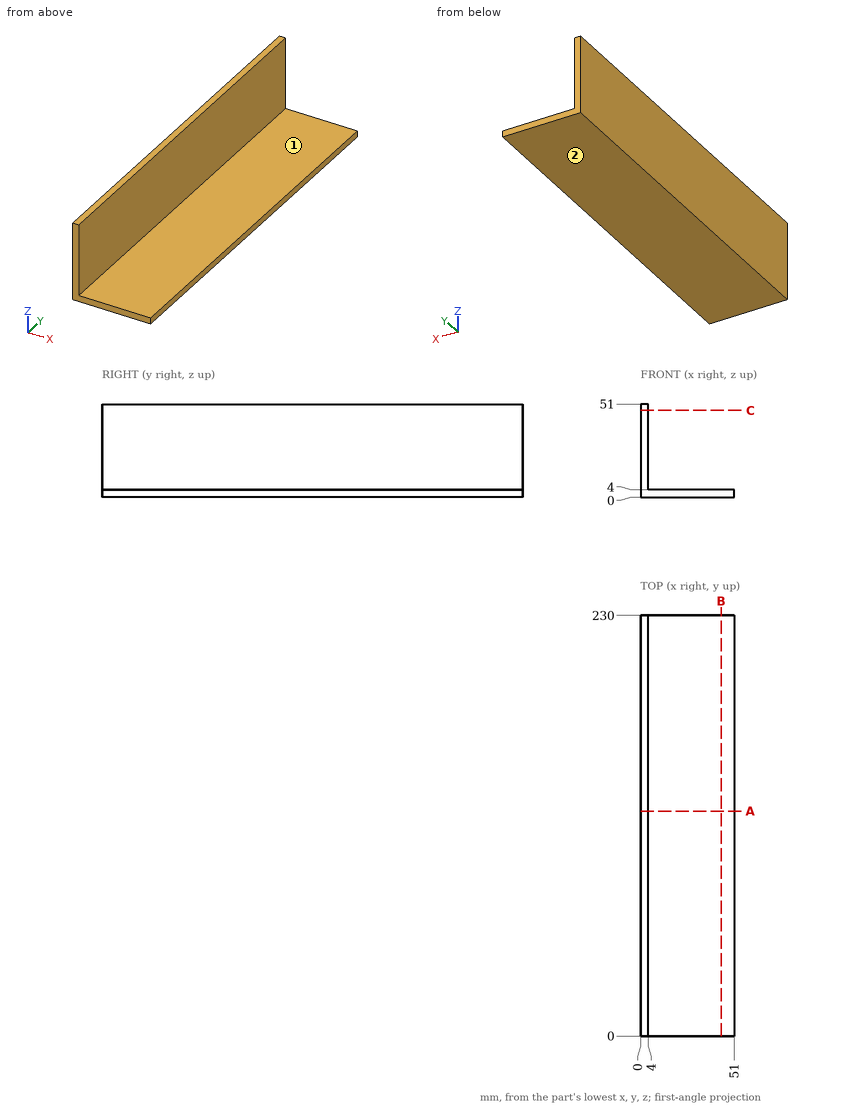
Study the drawing (mm; zero at the part's minimum x, y, z) and answer. A direction names the side the tool comes from. Coordinates: 2 decimals unless noted, no trailing zeros. Write each loop counter-clockwise with the first axis right and the second up, starting at its lowest first coordinate (ties: lowest second). Pieces come first, ordered by that corner, then holes.
Q1. A cutting plane is placed at A-A, the plane y = 123. Give the vertices of the cut face in (x, z), then the cut area to 3 significant figures.
Q2. Which of the six approach directions +Z, -Z, +X, -X, +Y, -Y give full straight-line access (tool end or side, diameter ignored) to the marked faces 1 and 2?
Q3. This flat-tipped pin is pushed along its axis until it touches: pin 1 Ø10 at (y, z) = (201, 32.5) entering from +X. Where does it stop, or does it pass through?
Q4. Find the intervals of material crossed by line 1 (X direction, y = 28, z = 45.5), in increasing order.
Q5. A cutting plane is placed at C-C, the plane z = 47.5. Give the vertices of the cut face in (x, y), then the cut area to 3 significant figures.
Q6. A cutting plane is placed at B-B, the plane x = 44. Give the vertices of the cut face in (y, z).
Findings below:
1. outline: (0, 0) - (51, 0) - (51, 4) - (4, 4) - (4, 51) - (0, 51) - close
1. area: 392 mm2
2. face 1: +Z, +X, +Y, -Y
2. face 2: -Z, +X, -X, +Y, -Y
3. pin 1: stops at x = 4
4. line 1: x = 0 to 4
5. outline: (0, 0) - (4, 0) - (4, 230) - (0, 230) - close
5. area: 920 mm2
6. outline: (0, 0) - (230, 0) - (230, 4) - (0, 4) - close
